```python
from build123d import *

# Parameters (mm, degrees)
F1_DEPTH = 3
F3_DEPTH = 25


with BuildPart() as f1:
    # F0 (on Top) → F1 (new body)
    with BuildSketch(Plane.XY):
        Polygon((31.2, 0), (0, 0), (0, -30.118711), (-8.601577, -30.118711), (-8.601577, -63.583943), (0, -63.583943), (0, -94.037309), (73.053598, -94.037309), (73.053598, -81.655175), (100.2, -81.655175), (100.2, -95.087759), (171.5, -95.087759), (171.5, -77.062562), (200.4, -77.062562), (200.4, -95.087759), (265.7, -95.087759), (265.7, -39.6), (271.7, -39.6), (271.7, -10), (231.6, -10), (231.6, 0), (200.4, 0), (200.4, -39.2), (171.5, -39.2), (171.5, -10), (131.4, -10), (131.4, 0), (100.2, 0), (100.2, -39.2), (71.3, -39.2), (71.3, -10), (31.2, -10), align=None)
    extrude(amount=F1_DEPTH)

    # F2 (on face) → F3 (join)
    with BuildSketch(Plane.XY.offset(3)):
        Polygon((31.2, -10), (31.2, 0), (0, 0), (0, -30.118711), (-8.601577, -30.118711), (-8.601577, -63.583943), (0, -63.583943), (0, -94.037309), (73.053598, -94.037309), (73.053598, -81.655175), (100.2, -81.655175), (100.2, -95.087759), (171.5, -95.087759), (171.5, -77.062562), (200.4, -77.062562), (200.4, -95.087759), (265.7, -95.087759), (265.7, -39.6), (271.7, -39.6), (271.7, -10), (231.6, -10), (231.6, 0), (200.4, 0), (200.4, -39.2), (171.5, -39.2), (171.5, -10), (131.4, -10), (131.4, 0), (100.2, 0), (100.2, -39.2), (71.3, -39.2), (71.3, -10), align=None)
        Polygon((3, -91.037309), (3, -60.583943), (-5.601577, -60.583943), (-5.601577, -33.118711), (3, -33.118711), (3, -3), (28.2, -3), (28.2, -13), (68.3, -13), (68.3, -42.2), (103.2, -42.2), (103.2, -3), (128.4, -3), (128.4, -13), (168.5, -13), (168.5, -42.2), (203.4, -42.2), (203.4, -3), (228.6, -3), (228.6, -13), (268.7, -13), (268.7, -36.6), (262.7, -36.6), (262.7, -92.087759), (203.4, -92.087759), (203.4, -74.062562), (168.5, -74.062562), (168.5, -92.087759), (103.2, -92.087759), (103.2, -78.655175), (70.053598, -78.655175), (70.053598, -91.037309), align=None, mode=Mode.SUBTRACT)
    extrude(amount=F3_DEPTH)


solid = f1.part
```
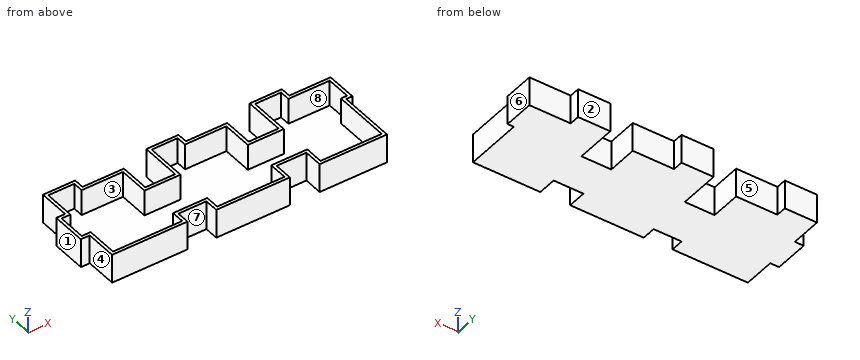
The model under review builds one solid part; all positions refer to its coordinate system, in mm. Face numbers are marked on the shaded views. A direction names the side the tool comes from. Coordinates: 2 decimals unless noted, no trailing zeros. Write each loop counter-clockwise with the first axis right and the second up, starting at its lowest first coordinate (ties: lowest second). Pieces come first, ordered by that corner, then holes. Notation, with made-up numbers: (54, 50.5) -> (58, 50.5) arc R33 cw to (58, 83.5) -> close; hole circle Ø9 at (9, -39). An arc over 180 degrees is marked (long way). One line per item, written item: value. Start each with the question number.
Q1. Add section D-D, the plane y = -6. Give the boundary of the cut face in (x, z), then the cut area to 3 significant figures.
Q2. Add section B-B, the plane x = 88.5. Give the boundary of the cut face in (y, z), then the cut area to 3 significant figures.
Q3. To check wall thickness, follow probe 1 along X at (y, z) = (-37.5, 23); probe 2 along X at (y, z) = (-89, 4); probe 3 along X at (y, z) = (-77, 13.5). State the ranges of each line that lie inside material, in increasing order.
Q4. Clearance check with flat-ended pins moving along their axes: P1, Ø8.5, axis at y = -9, z = 15.5, coming from the -X side; P2, Ø3, axis at x = 157, z = 21.5, coming from the +Y side; P3, Ø8.5, axis at x = 28, z = 11.5, coming from the -Y side. State where each tip first meets the part, or that it passes through.
Q5. The part is to be moulded in two halves that separate along X. For the marked faces 1, 2 and 3, say which applies: +X half, -X half, draft (parallel to the pull), parting line (faces both ways), or undercut.
Q6. Add section C-C, the plane y = -53. Give the boundary of the cut face in (x, z).
Q7. For the marked faces 4, 5, 6, 7 and 8, list the 3-axis set-ups (+Z, -Z, +X, -X, +Y, -Y) from which the entire face can be reached by the end or side of a thin tool; tool diameter is ignored.
Q8. Add section A-A, the plane y = -22. Give the boundary of the cut face in (x, z).
Response:
1. outline: (0, 0) -> (31.2, 0) -> (31.2, 28) -> (28.2, 28) -> (28.2, 3) -> (3, 3) -> (3, 28) -> (0, 28) -> close; (100.2, 0) -> (131.4, 0) -> (131.4, 28) -> (128.4, 28) -> (128.4, 3) -> (103.2, 3) -> (103.2, 28) -> (100.2, 28) -> close; (200.4, 0) -> (231.6, 0) -> (231.6, 28) -> (228.6, 28) -> (228.6, 3) -> (203.4, 3) -> (203.4, 28) -> (200.4, 28) -> close
1. area: 731 mm²
2. outline: (-81.66, 0) -> (-39.2, 0) -> (-39.2, 28) -> (-42.2, 28) -> (-42.2, 3) -> (-78.66, 3) -> (-78.66, 28) -> (-81.66, 28) -> close
2. area: 277 mm²
3. probe 1: -8.6 to -5.6, 68.3 to 71.3, 100.2 to 103.2, 168.5 to 171.5, 200.4 to 203.4, 262.7 to 271.7
3. probe 2: 0 to 3, 70.05 to 73.05, 100.2 to 103.2, 168.5 to 171.5, 200.4 to 203.4, 262.7 to 265.7
3. probe 3: 0 to 3, 168.5 to 203.4, 262.7 to 265.7
4. P1: x = 0
4. P2: y = -10
4. P3: y = -94.04
5. face 1: -X half
5. face 2: draft
5. face 3: undercut
6. outline: (-8.6, 0) -> (265.7, 0) -> (265.7, 28) -> (262.7, 28) -> (262.7, 3) -> (-5.6, 3) -> (-5.6, 28) -> (-8.6, 28) -> close
7. face 4: +Z, -Z, -X, -Y
7. face 5: +Z, -Z, +Y
7. face 6: +Z, -Z, +X, +Y, -Y
7. face 7: +Z, -Z, -Y
7. face 8: +Z
8. outline: (0, 0) -> (71.3, 0) -> (71.3, 28) -> (68.3, 28) -> (68.3, 3) -> (3, 3) -> (3, 28) -> (0, 28) -> close; (100.2, 0) -> (171.5, 0) -> (171.5, 28) -> (168.5, 28) -> (168.5, 3) -> (103.2, 3) -> (103.2, 28) -> (100.2, 28) -> close; (200.4, 0) -> (271.7, 0) -> (271.7, 28) -> (268.7, 28) -> (268.7, 3) -> (203.4, 3) -> (203.4, 28) -> (200.4, 28) -> close
